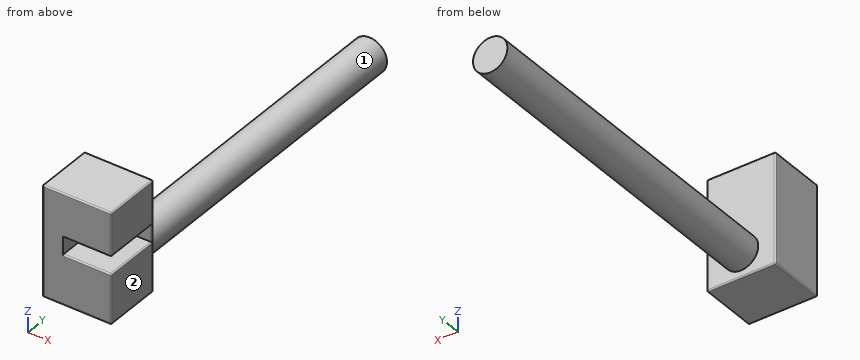
from build123d import *

# Parameters (mm, degrees)
SKETCH1_W           = 100
SKETCH1_H           = 160
BOSS_EXTRUDE1_DEPTH = 85
SKETCH2_R           = 25
BOSS_EXTRUDE2_DEPTH = 590
SKETCH3_W           = 25
SKETCH3_H           = 82
CUT_EXTRUDE1_DEPTH  = 70
FILLET2_R           = 2
FILLET3_R           = 5
FILLET4_R           = 2


with BuildPart() as part:
    # Sketch1 → Boss-Extrude1 (new body)
    with BuildSketch(Plane(origin=(0, 0, 0), x_dir=(1, 0, 0), z_dir=(0, 1, 0))):
        with Locations((-10.009659714, -61.441979522)):
            Rectangle(SKETCH1_W, SKETCH1_H)
    extrude(amount=BOSS_EXTRUDE1_DEPTH)

    # Sketch2 → Boss-Extrude2 (add)
    with BuildSketch(Plane(origin=(0, 0, 0), x_dir=(1, 0, 0), z_dir=(0, 1, 0))):
        with Locations(Location((-10.009659714, -16.441979522, 0), (0, 0, 270))):
            Circle(SKETCH2_R)
    extrude(amount=BOSS_EXTRUDE2_DEPTH)

    # Sketch3 → Cut-Extrude1 (cut)
    with BuildSketch(Plane(origin=(39.990340286, 0, 0), x_dir=(0, 0, -1), z_dir=(1, 0, 0))):
        with Locations((-66.178079743, 41)):
            Rectangle(SKETCH3_W, SKETCH3_H)
    extrude(amount=-CUT_EXTRUDE1_DEPTH, mode=Mode.SUBTRACT)

    # Fillet2
    fillet2_edges = [part.edges().sort_by_distance(p)[0] for p in [
        (39.990340286, 41, 53.678079743),
        (39.990340286, 82, 66.178079743),
        (39.990340286, 41, 78.678079743),
    ]]
    fillet(fillet2_edges, radius=FILLET2_R)

    # Fillet3
    fillet3_edges = [part.edges().sort_by_distance(p)[0] for p in [
        (-30.009659714, 82, 66.178079743),
    ]]
    fillet(fillet3_edges, radius=FILLET3_R)

    # Fillet4
    # the kernel refuses this fillet: 2 mm, written as the material it takes off along each edge
    with BuildSketch(Plane(origin=(-58.009659714, 83, -16.558020478), x_dir=(0, 0, -1), z_dir=(-1, 0, 0))) as fillet4_piece_1_section:
        Polygon((0, 0), (FILLET4_R, 0), (FILLET4_R, -FILLET4_R), (0, -FILLET4_R), align=None)
    fillet4_piece_1 = extrude(amount=FILLET4_R, mode=Mode.PRIVATE)
    fillet4_piece_1 = fillet4_piece_1 - Plane(origin=(-58.009659714, 83, -16.558020478), x_dir=(0, -0.7071067811865475, 0.7071067811865475), z_dir=(-1, 0, 0)) * Sphere(FILLET4_R, mode=Mode.PRIVATE)
    add(fillet4_piece_1, mode=Mode.SUBTRACT)
    with BuildSketch(Plane(origin=(37.990340286, 83, -16.558020478), x_dir=(0, 1, 0), z_dir=(0, 0, -1))) as fillet4_piece_2_section:
        Polygon((0, 0), (FILLET4_R, 0), (FILLET4_R, FILLET4_R), (0, FILLET4_R), align=None)
    fillet4_piece_2 = extrude(amount=FILLET4_R, mode=Mode.PRIVATE)
    fillet4_piece_2 = fillet4_piece_2 - Plane(origin=(37.990340286, 83, -16.558020478), x_dir=(-0.7071067811865475, -0.7071067811865475, 0), z_dir=(0, 0, -1)) * Sphere(FILLET4_R, mode=Mode.PRIVATE)
    add(fillet4_piece_2, mode=Mode.SUBTRACT)
    with BuildSketch(Plane(origin=(-58.009659714, 2, -16.558020478), x_dir=(0, 0, -1), z_dir=(-1, 0, 0))) as fillet4_piece_3_section:
        Polygon((0, 0), (FILLET4_R, 0), (FILLET4_R, FILLET4_R), (0, FILLET4_R), align=None)
    fillet4_piece_3 = extrude(amount=FILLET4_R, mode=Mode.PRIVATE)
    fillet4_piece_3 = fillet4_piece_3 - Plane(origin=(-58.009659714, 2, -16.558020478), x_dir=(0, 0.7071067811865475, 0.7071067811865475), z_dir=(-1, 0, 0)) * Sphere(FILLET4_R, mode=Mode.PRIVATE)
    add(fillet4_piece_3, mode=Mode.SUBTRACT)
    with BuildSketch(Plane(origin=(37.990340286, 2, -16.558020478), x_dir=(0, -1, 0), z_dir=(0, 0, -1))) as fillet4_piece_4_section:
        Polygon((0, 0), (FILLET4_R, 0), (FILLET4_R, -FILLET4_R), (0, -FILLET4_R), align=None)
    fillet4_piece_4 = extrude(amount=FILLET4_R, mode=Mode.PRIVATE)
    fillet4_piece_4 = fillet4_piece_4 - Plane(origin=(37.990340286, 2, -16.558020478), x_dir=(-0.7071067811865475, 0.7071067811865475, 0), z_dir=(0, 0, -1)) * Sphere(FILLET4_R, mode=Mode.PRIVATE)
    add(fillet4_piece_4, mode=Mode.SUBTRACT)
    with BuildSketch(Plane(origin=(37.990340286, 2, 139.441979522), x_dir=(0, -1, 0), z_dir=(0, 0, 1))) as fillet4_piece_5_section:
        Polygon((0, 0), (FILLET4_R, 0), (FILLET4_R, FILLET4_R), (0, FILLET4_R), align=None)
    fillet4_piece_5 = extrude(amount=FILLET4_R, mode=Mode.PRIVATE)
    fillet4_piece_5 = fillet4_piece_5 - Plane(origin=(37.990340286, 2, 139.441979522), x_dir=(-0.7071067811865475, 0.7071067811865475, 0), z_dir=(0, 0, 1)) * Sphere(FILLET4_R, mode=Mode.PRIVATE)
    add(fillet4_piece_5, mode=Mode.SUBTRACT)
    with BuildSketch(Plane(origin=(37.990340286, 83, 139.441979522), x_dir=(0, 1, 0), z_dir=(0, 0, 1))) as fillet4_piece_6_section:
        Polygon((0, 0), (FILLET4_R, 0), (FILLET4_R, -FILLET4_R), (0, -FILLET4_R), align=None)
    fillet4_piece_6 = extrude(amount=FILLET4_R, mode=Mode.PRIVATE)
    fillet4_piece_6 = fillet4_piece_6 - Plane(origin=(37.990340286, 83, 139.441979522), x_dir=(-0.7071067811865475, -0.7071067811865475, 0), z_dir=(0, 0, 1)) * Sphere(FILLET4_R, mode=Mode.PRIVATE)
    add(fillet4_piece_6, mode=Mode.SUBTRACT)
    with BuildSketch(Plane(origin=(-58.009659714, 83, 139.441979522), x_dir=(-1, 0, 0), z_dir=(0, 0, 1))) as fillet4_piece_7_section:
        Polygon((0, 0), (FILLET4_R, 0), (FILLET4_R, -FILLET4_R), (0, -FILLET4_R), align=None)
    fillet4_piece_7 = extrude(amount=FILLET4_R, mode=Mode.PRIVATE)
    fillet4_piece_7 = fillet4_piece_7 - Plane(origin=(-58.009659714, 83, 139.441979522), x_dir=(0.7071067811865475, -0.7071067811865475, 0), z_dir=(0, 0, 1)) * Sphere(FILLET4_R, mode=Mode.PRIVATE)
    add(fillet4_piece_7, mode=Mode.SUBTRACT)
    with BuildSketch(Plane(origin=(-58.009659714, 2, 139.441979522), x_dir=(-1, 0, 0), z_dir=(0, 0, 1))) as fillet4_piece_8_section:
        Polygon((0, 0), (FILLET4_R, 0), (FILLET4_R, FILLET4_R), (0, FILLET4_R), align=None)
    fillet4_piece_8 = extrude(amount=FILLET4_R, mode=Mode.PRIVATE)
    fillet4_piece_8 = fillet4_piece_8 - Plane(origin=(-58.009659714, 2, 139.441979522), x_dir=(0.7071067811865475, 0.7071067811865475, 0), z_dir=(0, 0, 1)) * Sphere(FILLET4_R, mode=Mode.PRIVATE)
    add(fillet4_piece_8, mode=Mode.SUBTRACT)
    with BuildSketch(Plane(origin=(37.990340286, 0, 53.678079743), x_dir=(0, 0, -1), z_dir=(-1, 0, 0)), Plane(origin=(37.990340286, 0, 78.678079743), x_dir=(0, 1, 0), z_dir=(-1, 0, 0))) as fillet4_piece_9:
        with BuildLine():
            CenterArc((FILLET4_R, -FILLET4_R), FILLET4_R, 90, 90)
            Line((0, -FILLET4_R), (0, 0))
            Line((0, 0), (FILLET4_R, 0))
        make_face()
    extrude(amount=68, mode=Mode.SUBTRACT)
    with BuildSketch(Plane(origin=(37.990340286, 0, 51.678079743), x_dir=(1, 0, 0), z_dir=(0, 0, -1))) as fillet4_piece_10:
        with BuildLine():
            CenterArc((2 - FILLET4_R, -FILLET4_R), FILLET4_R, 0, 90)
            Line((2, -FILLET4_R), (2, 0))
            Line((2, 0), (2 - FILLET4_R, 0))
        make_face()
    revolve(axis=Axis((37.990340286, 0, 51.678079743), (0, -1, 0)), revolution_arc=90, mode=Mode.SUBTRACT)
    with BuildSketch(Plane(origin=(37.990340286, 0, 80.678079743), x_dir=(1, 0, 0), z_dir=(0, 0, 1))) as fillet4_piece_11:
        with BuildLine():
            CenterArc((2 - FILLET4_R, FILLET4_R), FILLET4_R, 270, 90)
            Line((2, FILLET4_R), (2, 0))
            Line((2, 0), (2 - FILLET4_R, 0))
        make_face()
    revolve(axis=Axis((37.990340286, 0, 80.678079743), (0, 1, 0)), revolution_arc=90, mode=Mode.SUBTRACT)
    with BuildSketch(Plane(origin=(-58.009659714, 85, -18.558020478), x_dir=(0, -1, 0), z_dir=(1, 0, 0)), Plane(origin=(-58.009659714, 0, -18.558020478), x_dir=(0, 0, 1), z_dir=(1, 0, 0)), Plane(origin=(37.990340286, 85, 141.441979522), x_dir=(0, -1, 0), z_dir=(-1, 0, 0)), Plane(origin=(37.990340286, 0, 141.441979522), x_dir=(0, 0, -1), z_dir=(-1, 0, 0))) as fillet4_piece_12:
        with BuildLine():
            CenterArc((FILLET4_R, -FILLET4_R), FILLET4_R, 90, 90)
            Line((0, -FILLET4_R), (0, 0))
            Line((0, 0), (FILLET4_R, 0))
        make_face()
    extrude(amount=96, mode=Mode.SUBTRACT)
    with BuildSketch(Plane(origin=(-60.009659714, 2, -18.558020478), x_dir=(0, 0, 1), z_dir=(0, 1, 0)), Plane(origin=(39.990340286, 2, 141.441979522), x_dir=(0, 0, -1), z_dir=(0, 1, 0)), Plane(origin=(-60.009659714, 2, 141.441979522), x_dir=(1, 0, 0), z_dir=(0, 1, 0))) as fillet4_piece_13:
        with BuildLine():
            CenterArc((FILLET4_R, FILLET4_R), FILLET4_R, 180, 90)
            Line((0, FILLET4_R), (0, 0))
            Line((0, 0), (FILLET4_R, 0))
        make_face()
    extrude(amount=81, mode=Mode.SUBTRACT)
    with BuildSketch(Plane(origin=(39.990340286, 0, -16.558020478), x_dir=(-1, 0, 0), z_dir=(0, 0, 1))) as fillet4_piece_14:
        with BuildLine():
            CenterArc((FILLET4_R, -FILLET4_R), FILLET4_R, 90, 90)
            Line((0, -FILLET4_R), (0, 0))
            Line((0, 0), (FILLET4_R, 0))
        make_face()
    extrude(amount=68.236100221, mode=Mode.SUBTRACT)
    with BuildSketch(Plane(origin=(39.990340286, 0, 80.678079743), x_dir=(-1, 0, 0), z_dir=(0, 0, 1))) as fillet4_piece_15:
        with BuildLine():
            CenterArc((FILLET4_R, -FILLET4_R), FILLET4_R, 90, 90)
            Line((0, -FILLET4_R), (0, 0))
            Line((0, 0), (FILLET4_R, 0))
        make_face()
    extrude(amount=58.763899779, mode=Mode.SUBTRACT)
    with BuildSketch(Plane(origin=(39.990340286, 2, -18.558020478), x_dir=(0, 0, 1), z_dir=(0, 1, 0))) as fillet4_piece_16:
        with BuildLine():
            CenterArc((FILLET4_R, -FILLET4_R), FILLET4_R, 90, 90)
            Line((0, -FILLET4_R), (0, 0))
            Line((0, 0), (FILLET4_R, 0))
        make_face()
    extrude(amount=81, mode=Mode.SUBTRACT)
    with BuildSketch(Plane(origin=(39.990340286, 85, -16.558020478), x_dir=(0, -1, 0), z_dir=(0, 0, 1)), Plane(origin=(-60.009659714, 0, 139.441979522), x_dir=(1, 0, 0), z_dir=(0, 0, -1)), Plane(origin=(-60.009659714, 85, 139.441979522), x_dir=(0, -1, 0), z_dir=(0, 0, -1))) as fillet4_piece_17:
        with BuildLine():
            CenterArc((FILLET4_R, -FILLET4_R), FILLET4_R, 90, 90)
            Line((0, -FILLET4_R), (0, 0))
            Line((0, 0), (FILLET4_R, 0))
        make_face()
    extrude(amount=156, mode=Mode.SUBTRACT)


solid = part.part
Check sheet for the modelled part. Datum: model origin and axes. Units: mm. Face numbers are marked on the shaded views. A direction names the side the tool comes from. Round coordinates to 2 decimals unless told otherwise and drop trailing zeros. Write each loop counter-clockwise with the first axis right and the second up, starting at its lowest first coordinate (ties: lowest second). Pieces come first, ordered by that corner, then holes. Notation, with made-up numbers: (45, 37) -> (71, 37) arc R23 ccw to (71, 61) -> close; hole circle Ø9 at (-10.75, -7). An arc over 180 degrees is marked (long way). Answer as CSV lines item,"result". Start each with the question number.
1) Material ranges on line 1 (Y direction, x = -25, z = 112); line 2 (Z direction, x = -10, y = 444.5); line 3 (Y direction, x = 26, z = 63.5), recorded low to high. Write a range as from..to.
2) Section check A-A on x = 31. Enter the section's corners in (y, z).
3) Section check C-C on y = 474. Enter the section's corners in (x, z).
4) Go/stop test with flat-tipped pins: P1, Ø8, axis at x = -2.5, y = 346.5, coming from the -Z side; P2, Ø8, axis at x = 20.5, z = 52.5, coming from the +Y side; P3, Ø4, axis at x = 0, y = 110, coming from the +Z side. Record where each tip stops, or that it passes through.
5) Tool access check on the marked faces 1 and 2. Record the directions out of +Z, -Z, +X, -X, +Y, -Y that give a thin tool (end or side, any length) a straight path to the whole face; none if there is none.
6) Section check D-D on x = 5. Enter the section's corners in (y, z), and give its area (3 significant figures).
7) Section check B-B on z = 16.5. Enter the section's corners in (x, y).
Found:
1,line 1,"y = 0..85"
1,line 2,"z = -8.56..41.44"
1,line 3,"y = 82..85"
2,outline,"(0, -16.56) arc R2 ccw to (2, -18.56) -> (83, -18.56) arc R2 ccw to (85, -16.56) -> (85, 139.44) arc R2 ccw to (83, 141.44) -> (2, 141.44) arc R2 ccw to (0, 139.44) -> (0, 80.68) arc R2 ccw to (2, 78.68) -> (82, 78.68) -> (82, 53.68) -> (2, 53.68) arc R2 ccw to (0, 51.68) -> close"
3,outline,"circle Ø50 at (-10.01, 16.44)"
4,P1,"stops at z = -8.31"
4,P2,"stops at y = 85"
4,P3,"stops at z = 40.12"
5,face 1,"+Y"
5,face 2,"+Z, -Z, +X, +Y, -Y"
6,outline,"(0, -16.56) arc R2 ccw to (2, -18.56) -> (83, -18.56) arc R2 ccw to (85, -16.56) -> (85, -3.55) -> (590, -3.55) -> (590, 36.43) -> (85, 36.43) -> (85, 139.44) arc R2 ccw to (83, 141.44) -> (2, 141.44) arc R2 ccw to (0, 139.44) -> (0, 80.68) arc R2 ccw to (2, 78.68) -> (82, 78.68) -> (82, 53.68) -> (2, 53.68) arc R2 ccw to (0, 51.68) -> close"
6,area,"31,700 mm^2"
7,outline,"(-60.01, 2) arc R2 ccw to (-58.01, 0) -> (37.99, 0) arc R2 ccw to (39.99, 2) -> (39.99, 83) arc R2 ccw to (37.99, 85) -> (14.99, 85) -> (14.99, 590) -> (-35.01, 590) -> (-35.01, 85) -> (-58.01, 85) arc R2 ccw to (-60.01, 83) -> close"
